from build123d import *

# Parameters (mm, degrees)
BOSS_EXTRUDE1_DEPTH = 2
BOSS_EXTRUDE2_DEPTH = 6
SKETCH24_R          = 3.9
BOSS_EXTRUDE5_DEPTH = 2.3
SKETCH30_W          = 2.408612022
SKETCH30_H          = 1.324178481
CUT_EXTRUDE12_DEPTH = 8
FILLET2_R           = 2
CUT_EXTRUDE11_DEPTH = 10


with BuildPart() as part:
    # Sketch2 → Boss-Extrude1 (new body)
    with BuildSketch(Plane.XY):
        with BuildLine():
            Line((-2.5, 7.5), (-20.7, 7.5))
            Line((-20.7, 7.5), (-20.7, -7.5))
            Line((-20.7, -7.5), (-6.7, -7.5))
            Line((-6.7, -7.5), (-4.2, -5.6))
            ThreePointArc((-4.2, -5.6), (3.130495168, -6.260990337), (7, 0))
            ThreePointArc((7, 0), (4.949747468, 4.949747468), (0, 7))
            Line((0, 7), (0, 7.5))
            Line((0, 7.5), (-2.5, 7.5))
        make_face()
    extrude(amount=BOSS_EXTRUDE1_DEPTH)

    # Sketch4 → Boss-Extrude2 (add)
    with BuildSketch(Plane.XY.offset(2)):
        Polygon((-20.7, -7.5), (-20.7, 7.5), (-0.7, 7.5), (0, 7.5), (0, 5.3), (-0.7, 5.3), (-6.7, 5.3), (-6.7, 2), (-19.5, 2), (-19.5, -6), (-6.759079174, -6), (-6.7, -7.5), (-19.292624541, -7.5), align=None)
    extrude(amount=BOSS_EXTRUDE2_DEPTH)

    # Sketch24 → Boss-Extrude5 (add)
    with BuildSketch(Plane.XY.offset(2)):
        Circle(SKETCH24_R)
    extrude(amount=BOSS_EXTRUDE5_DEPTH)

    # Sketch30 → Cut-Extrude12 (cut)
    with BuildSketch(Plane(origin=(-6.7, 0, 0), x_dir=(0, 0, -1), z_dir=(1, 0, 0))):
        with Locations((-3.261593395, 4.63791076)):
            Rectangle(SKETCH30_W, SKETCH30_H)
    extrude(amount=-CUT_EXTRUDE12_DEPTH, mode=Mode.SUBTRACT)

    # Fillet2
    fillet2_edges = [part.edges().sort_by_distance(p)[0] for p in [
        (-20.7, 0, 0),
        (-20.7, 7.5, 4),
        (-13.7, -7.5, 0),
        (-10.35, 7.5, 0),
        (-20.7, -7.5, 4),
    ]]
    fillet(fillet2_edges, radius=FILLET2_R)

    # Sketch28 → Cut-Extrude11 (cut)
    with BuildSketch(Plane.XY.offset(4.3)):
        with BuildLine():
            Line((-1, 1.656278148), (-1, -1.656278148))
            ThreePointArc((-1, -1.656278148), (1.934749933, 0), (-1, 1.656278148))
        make_face()
    extrude(amount=-CUT_EXTRUDE11_DEPTH, mode=Mode.SUBTRACT)


solid = part.part
For this review, take the finished solid that the model builds, in its own axes (mm). A direction names the side the tool comes from. Round coordinates to 2 decimals unless told otherwise and drop trailing zeros. Loops run counter-clockwise (first coordinate to the right, second up) from the corner with the lowest first, then second, coordinate; pieces in that order, holes last. Notation, with made-up numbers: (54.25, 75) - (87.25, 75) arc R16 cw to (87.25, 92) - close; hole circle Ø6 at (29, 66.25). An arc over 180 degrees is marked (long way). Put each result on its own line as item: value. Start each with the question number.
1. Mouldability with a two-part tool opening along Y and no side actions: class faces 1 (the cylindrical face through (-9.58, -6.63, 0.35)), 2 (the flat face through (-20.7, 0, 5)), 3 (the flat face through (-11, 5, 4.466)) as +Y half, -Y half, draft (parallel to the pull), parting line (faces both ways), or undercut.
2. Consider section C-C on z = 7.25. State the section outline as (x, y) points, plus the area to 3 significant figures.
3. Consider section D-D on y = 3.5. State the section outline as (x, z) points, plus the area to 3 significant figures.
4. For probe 1 along Y at (x, z) = (-8.5, 4); probe 2 along Z at (x, y) = (-9, -3); probe 3 along X at (y, z) = (-3.5, 6), list the stretches that pass through material, from the lowest coordinate up. Write a range as [from, to].
5. Insertion check: P1, Ø1, axis at x = 2, z = 4.5, coming from the +Y side; P2, Ø6, axis at x = 0, y = 1.5, coming from the +Z side; P3, Ø3, axis at x = -1.5, z = 6.5, coming from the -Y side. Each pin has a flat end and moves straight along its axis. Give the tip position at first contact, or say it passes through.
6. For faces 4 (the flat face through (-5.19, -6.35, 1.21)), 5 (the flat face through (-1, 0, 2)), 6 (the flat face through (0, 6, 5)), 7 (the flat face through (-6, 5.3, 4)), list the 3-axis set-ups (+Z, -Z, +X, -X, +Y, -Y) from which the entire face can be reached by the end or side of a thin tool; tool diameter is ignored.
7. Consider section A-A on z = 3. State the section outline as (x, y) points.
8. Consider section B-B on x = -13.5. State the section outline as (y, z) points.
Result sheet:
1. face 1: -Y half
1. face 2: draft
1. face 3: undercut
2. outline: (-20.7, -5.5) arc R2 ccw to (-18.7, -7.5) - (-6.7, -7.5) - (-6.76, -6) - (-19.5, -6) - (-19.5, 2) - (-6.7, 2) - (-6.7, 5.3) - (0, 5.3) - (0, 7.5) - (-18.7, 7.5) arc R2 ccw to (-20.7, 5.5) - close
2. area: 121 mm^2
3. outline: (-20.7, 2) arc R2 ccw to (-18.7, 0) - (6.06, 0) - (6.06, 2) - (1.72, 2) - (1.72, 4.3) - (-1.72, 4.3) - (-1.72, 2) - (-6.7, 2) - (-6.7, 8) - (-20.7, 8) - close
3. area: 145 mm^2
4. probe 1: [-7.5, -6], [2, 3.98], [5.3, 7.5]
4. probe 2: [0, 2]
4. probe 3: [-20.7, -19.5]
5. P1: y = 3.58
5. P2: z = 4.3
5. P3: y = 5.3
6. face 4: +Z, -Z, -Y
6. face 5: +Z, -Z
6. face 6: +Z, +X, +Y
6. face 7: +X
7. outline: (-20.7, -5.5) arc R2 ccw to (-18.7, -7.5) - (-6.7, -7.5) - (-6.76, -6) - (-19.5, -6) - (-19.5, 2) - (-6.7, 2) - (-6.7, 3.98) - (-14.7, 3.98) - (-14.7, 5.3) - (0, 5.3) - (0, 7.5) - (-18.7, 7.5) arc R2 ccw to (-20.7, 5.5) - close; circle Ø7.8 at (0, 0); hole (-1, -1.66) arc R1.93 ccw (long way) to (-1, 1.66) - close
8. outline: (-7.5, 2) arc R2 ccw to (-5.5, 0) - (5.5, 0) arc R2 ccw to (7.5, 2) - (7.5, 8) - (2, 8) - (2, 2) - (-6, 2) - (-6, 8) - (-7.5, 8) - close; hole (3.98, 2.06) - (5.3, 2.06) - (5.3, 4.47) - (3.98, 4.47) - close
